from build123d import *

# Parameters (mm, degrees)
BOSS_EXTRUDE1_DEPTH = 4.7752


with BuildPart() as part:
    # Sketch3 → Boss-Extrude1 (new body)
    with BuildSketch(Plane.XY):
        Polygon((10, 0), (10, 4.7752), (14.7752, 4.7752), (14.7752, 0), (25, 0), (35.2248, 0), (35.2248, 4.7752), (40, 4.7752), (40, 0), (50, 0), (50, 10), (45.2248, 10), (45.2248, 14.7752), (50, 14.7752), (50, 22.5), (50, 30.2248), (45.2248, 30.2248), (45.2248, 35), (50, 35), (50, 45), (40, 45), (40, 40.2248), (35.2248, 40.2248), (35.2248, 45), (14.7752, 45), (14.7752, 40.2248), (10, 40.2248), (10, 45), (0, 45), (0, 35), (4.7752, 35), (4.7752, 30.2248), (0, 30.2248), (0, 14.7752), (4.7752, 14.7752), (4.7752, 10), (0, 10), (0, 0), align=None)
    extrude(amount=-BOSS_EXTRUDE1_DEPTH)


solid = part.part
Can you work these out from the model? Positions are in its coordinate system, mm. A direction names the side the tool comes from. Give positions to 0.01 mm unless a question says otherwise; leave off trailing zeros. Order: outer loops, then holes, each group sorted by start corner. A loop starts at its lowest first (then second) coordinate and runs counter-clockwise, first axis right, second up. Notation, with made-up numbers: M -6.5,-13.75 L 31.5,-13.75 A15 ccw 31.5,15.25 Z; hole C -10.5,12.25 d6. An arc over 180 degrees is marked long. Use a Markdown table: item, result. Add a question column.
Item 1: Suppose I cut it at B-B (x = 46.5). List the corners of the cut face in (y, z) for me.
Item 2: Will these pins go through, and if not, where does the flat tip stop? pin 1 (1.4 mm diameter, centred on y = 33.5, z = -1.5, fed in from -X); pin 2 (1.4 mm diameter, centred on x = 13, z = -1.5, fed in from -Y).
Item 3: If I drill on L1, parallel to X at y = 42, z = -4.35; L2, parallel to Y at x = 3, z = -1.6; L3, parallel to X at y = 33.5, z = -3.7, over which ranges is the centre line in solid material (lowest first)? Write a range as [from, to].
Item 4: Suppose I cut it at A-A (y = 3). List the corners of the cut face in (x, z) for me.
Item 5: We'd pull the mould along X, two halves only. Please class faces 1 (the flat face through (12, 40.225, -2)), 2 (the flat face through (35.225, 43, -2)), 3 (the flat face through (45.225, 33, -2)), 4 (the flat face through (48, 30.225, -2)): +X half, -X half, draft (parallel to the pull), parting line (faces both ways), or undercut.
Item 6: For faces 5 (the flat face through (48, 10, -2)), 6 (the flat face through (12, 4.775, -2)), 7 (the flat face through (10, 43, -2)), which set-ups out of +Z, -Z, +X, -X, +Y, -Y let a thin tool reach every point of the face, with its end or its side?
Answer sheet:
| question | item | result |
|---|---|---|
| 1 | outline | M 0,-4.78 L 10,-4.78 L 10,0 L 0,0 Z; M 14.78,-4.78 L 30.22,-4.78 L 30.22,0 L 14.78,0 Z; M 35,-4.78 L 45,-4.78 L 45,0 L 35,0 Z |
| 2 | pin 1 | stops at x = 4.78 |
| 2 | pin 2 | stops at y = 4.78 |
| 3 | L1 | x = [0, 10], [14.78, 35.22], [40, 50] |
| 3 | L2 | y = [0, 10], [14.78, 30.22], [35, 45] |
| 3 | L3 | x = [4.78, 45.22] |
| 4 | outline | M 0,-4.78 L 10,-4.78 L 10,0 L 0,0 Z; M 14.78,-4.78 L 35.22,-4.78 L 35.22,0 L 14.78,0 Z; M 40,-4.78 L 50,-4.78 L 50,0 L 40,0 Z |
| 5 | face 1 | undercut |
| 5 | face 2 | undercut |
| 5 | face 3 | +X half |
| 5 | face 4 | draft |
| 6 | face 5 | +Z, -Z, +X |
| 6 | face 6 | +Z, -Z, -Y |
| 6 | face 7 | +Z, -Z, +Y |
